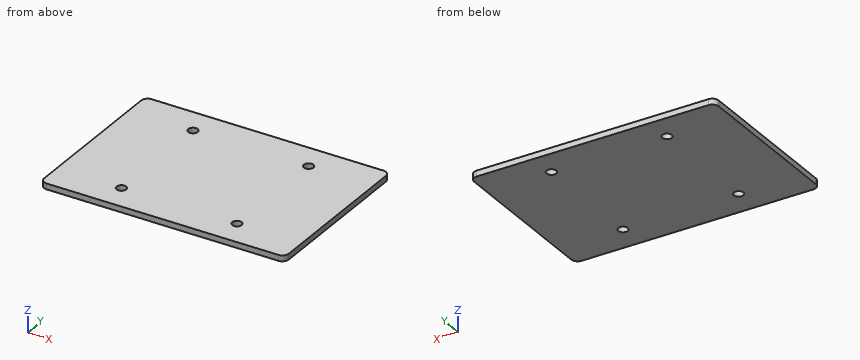
from build123d import *

# Parameters (mm, degrees)
SKETCH2_W           = 127
SKETCH2_H           = 88
BOSS_EXTRUDE1_DEPTH = 3
FILLET1_R           = 3.38
SKETCH3_R           = 2.5
CUT_EXTRUDE1_DEPTH  = 4


with BuildPart() as part:
    # Sketch2 → Boss-Extrude1 (new body)
    with BuildSketch(Plane.XY):
        Rectangle(SKETCH2_W, SKETCH2_H)
    extrude(amount=BOSS_EXTRUDE1_DEPTH)

    # Fillet1
    fillet1_edges = [part.edges().sort_by_distance(p)[0] for p in [
        (63.5, -44, 1.5),
        (-63.5, -44, 1.5),
        (-63.5, 44, 1.5),
        (63.5, 44, 1.5),
    ]]
    fillet(fillet1_edges, radius=FILLET1_R)

    # Sketch3 → Cut-Extrude1 (cut, through all)
    with BuildSketch(Plane(origin=(0, 0, 0), x_dir=(-1, 0, 0), z_dir=(0, 0, -1))):
        with Locations((-30, -30)):
            Circle(SKETCH3_R)
        with Locations((-30, 30)):
            Circle(SKETCH3_R)
        with Locations((30, 30)):
            Circle(SKETCH3_R)
        with Locations((30, -30)):
            Circle(SKETCH3_R)
    extrude(amount=-CUT_EXTRUDE1_DEPTH, mode=Mode.SUBTRACT)


solid = part.part
Design review of the part built by this model. Coordinates are the model's own, in mm. Coordinates: 2 decimals unless noted, no trailing zeros. Order: outer loops, then holes, each group sorted by start corner. A loop starts at its lowest first (then second) coordinate and runs counter-clockwise, first axis right, second up. Notation, with made-up numbers: M 24.5,-1.75 L 58.5,-1.75 A6 cw 58.5,9.25 Z; hole C 22,20 d9. An arc over 180 degrees is marked long. Use a Markdown table: item, result.
(1) Wall thickness on probe 1 along Y at (x, z) = (30, 1.9); probe 2 along Y at (x, z) = (28.5, 2.7); probe 3 along X at (y, z) = (31, 1.8): over which ranges is each line inside the solid? List them lowest first.
Worked answers:
| item | result |
|---|---|
| probe 1 | y = -44 to -32.5, -27.5 to 27.5, 32.5 to 44 |
| probe 2 | y = -44 to -32, -28 to 28, 32 to 44 |
| probe 3 | x = -63.5 to -32.29, -27.71 to 27.71, 32.29 to 63.5 |
(2) Add section B-B (y = -30). Give the boundary of the cut face in (x, z).
Worked answers:
| item | result |
|---|---|
| outline | M -63.5,0 L -32.5,0 L -32.5,3 L -63.5,3 Z; M -27.5,0 L 27.5,0 L 27.5,3 L -27.5,3 Z; M 32.5,0 L 63.5,0 L 63.5,3 L 32.5,3 Z |
(3) Add section A-A (x = 30). Give the boundary of the cut face in (y, z).
Worked answers:
| item | result |
|---|---|
| outline | M -44,0 L -32.5,0 L -32.5,3 L -44,3 Z; M -27.5,0 L 27.5,0 L 27.5,3 L -27.5,3 Z; M 32.5,0 L 44,0 L 44,3 L 32.5,3 Z |
